from build123d import *

# Parameters (mm, degrees)
SKETCH003_W  = 25.4
SKETCH003_H  = 25.4
PAD003_DEPTH = 2.1082
SKETCH004_R  = 1.651
POCKET_DEPTH = 2.1092
SKETCH005_R  = 7.747
PAD004_DEPTH = 15.9004
SKETCH006_R  = 7.747
PAD005_DEPTH = 3.598333
SKETCH007_R  = 1.4986
PAD006_DEPTH = 10.795


with BuildPart() as part:
    # Sketch003 → Pad003 (new body)
    with BuildSketch(Plane.XY):
        with Locations((12.7, 12.7)):
            Rectangle(SKETCH003_W, SKETCH003_H)
    extrude(amount=PAD003_DEPTH)

    # Sketch004 (on Face6 of Pad003) → Pocket (cut, through all)
    with BuildSketch(Plane.XY.offset(2.1082)):
        with Locations((3.5814, 21.8186)):
            Circle(SKETCH004_R)
        with Locations((21.8186, 21.8186)):
            Circle(SKETCH004_R)
        with Locations((21.8186, 3.5814)):
            Circle(SKETCH004_R)
        with Locations((3.5814, 3.5814)):
            Circle(SKETCH004_R)
    extrude(amount=-POCKET_DEPTH, mode=Mode.SUBTRACT)

    # Sketch005 → Pad004 (join)
    with BuildSketch(Plane.XY):
        with Locations((12.7, 12.7)):
            Circle(SKETCH005_R)
    extrude(amount=PAD004_DEPTH)

    # Sketch006 → Pad005 (join)
    with BuildSketch(Plane.XY):
        with Locations((12.7, 12.7)):
            Circle(SKETCH006_R)
    extrude(amount=-PAD005_DEPTH)

    # Sketch007 → Pad006 (join)
    with BuildSketch(Plane.XY):
        with Locations((12.7, 12.7)):
            Circle(SKETCH007_R)
    extrude(amount=-PAD006_DEPTH)


with BuildPart() as part_1:
    # Body001 placement: moved
    add(part.part.moved(Location((35.56, 0, 0))))


solid = part_1.part
Geometry check sheet. Reference: the model listing, model coordinates, mm. A direction names the side the tool comes from. Give positions to 0.01 mm unless a question says otherwise; leave off trailing zeros. Loops run counter-clockwise (first coordinate to the right, second up) from the corner with the lowest first, then second, coordinate; pieces in that order, holes last.
(1) Set-up check for faces 1 (the cylindrical face through (42.55, 17.936, -1.774)), 2 (the flat face through (48, 13, 15.9)), 3 (the cylindrical face through (42.55, 17.936, 8.908)): record each of +Z, -Z, +X, -X, +Y, -Y from which the full face is reachable in a straight line by a thin tool's end or side.
From the geometry:
face 1: -Z
face 2: +Z, +X, -X, +Y, -Y
face 3: +Z
(2) Depth check by flat-ended pin: pin 1 Ø10 at (x, z) = (53.5, 8.5) entering from +Y; pin 2 Ø5.5 at (x, y) = (39.14, 21.82) entering from -Z; pin 3 Ø1.5 at (x, y) = (55, 7) entering from +Z; pin 4 Ø2 at (x, z) = (58.5, -3.5) entering from -Y. Enter the tip coordinate at first touch or a pass-through.
From the geometry:
pin 1: stops at y = 20.44
pin 2: stops at z = 0
pin 3: stops at z = 2.11
pin 4: passes through
(3) Section check B-B on y = 12.7. Record the cut outline in (x, z) (3 decimals), then the cut area to 3 significant figures.
From the geometry:
outline: (35.56, 0) - (40.513, 0) - (40.513, -3.598) - (46.761, -3.598) - (46.761, -10.795) - (49.759, -10.795) - (49.759, -3.598) - (56.007, -3.598) - (56.007, 0) - (60.96, 0) - (60.96, 2.108) - (56.007, 2.108) - (56.007, 15.9) - (40.513, 15.9) - (40.513, 2.108) - (35.56, 2.108) - close
area: 345 mm2
(4) Thickness scan on L1, parallel to X at y = 13, z = 5; L2, parallel to Z at x = 44.75, y = 8.75; L3, parallel to Z at x = 55.25, y = 8.75. Record the ranges inside material, lowest first.
From the geometry:
L1: x = 40.52 to 56
L2: z = -3.6 to 15.9
L3: z = 0 to 2.11
(5) Section check D-D on z = -1.25. Record the cut outline in (x, y), then the cut area to 3 significant figures.
From the geometry:
outline: circle Ø15.49 at (48.26, 12.7)
area: 189 mm2
(6) Release check for a two-part mould opening along X. For faces 4 (the cylindrical face through (40.667, 2.949, 1.069)), 5 (the flat face through (35.56, 13, 1)), 6 (the flat face through (42, 19, 0)) record: released by +X, released by -X, zero draft, split by the parting line, or undercut.
From the geometry:
face 4: undercut
face 5: released by -X
face 6: zero draft
(7) Section check A-A on x = 48.26. Record the cut outline in (y, z) (3 decimals), then the cut area to 3 significant figures.
From the geometry:
outline: (0, 0) - (4.953, 0) - (4.953, -3.598) - (11.201, -3.598) - (11.201, -10.795) - (14.199, -10.795) - (14.199, -3.598) - (20.447, -3.598) - (20.447, 0) - (25.4, 0) - (25.4, 2.108) - (20.447, 2.108) - (20.447, 15.9) - (4.953, 15.9) - (4.953, 2.108) - (0, 2.108) - close
area: 345 mm2
(8) Section check C-C on x = 39.25. Record the cut outline in (y, z).
From the geometry:
outline: (0, 0) - (1.93, 0) - (1.93, 2.11) - (0, 2.11) - close; (5.23, 0) - (20.17, 0) - (20.17, 2.11) - (5.23, 2.11) - close; (23.47, 0) - (25.4, 0) - (25.4, 2.11) - (23.47, 2.11) - close
